Can you work these out from the model? Positions are in its coordinate system, mm. Face numbers are marked on the shaded views. A direction names the side the tool comes from. Round coordinates to 2 decimals unless told otherwise and drop trailing zeros. Write each loop counter-clockwise with the first axis right and the second up, starting at its lowest first coordinate (ties: lowest second). Pieces come first, ordered by that corner, then holes. Notation, with made-up numbers: M 69.5,82 L 95.5,82 A4 cw 95.5,88 Z; hole C 36,-20 d6. An arc over 180 degrees is marked long. Answer as a JSON object with one key per item and string values. Group by question number.
1) Suppose I cut it at C-C, the plane z = -9.5. Write out the boundary of the cut face in (x, y).
2) Suppose I cut it at B-B, the plane y = 0. State how many separate pieces and enclosed holes the cut face has, and give its area (3 significant figures).
3) Suppose I cut it at A-A, the plane z = -14.5. Write out the boundary of the cut face in (x, y).
4) If we mould it in two halves opening along X, with no side actions, what happens to the marked faces 4, 5 and 6? For each: +X half, -X half, draft (parallel to the pull), parting line (faces both ways), or undercut.
5) Please list where these lines run through material, in increasing order: L1, parallel to Y at x = 0, z = -21.25; L2, parallel to Z at x = 23, y = 13; L3, parallel to Y at x = -23.5, z = -29. Write a range as [from, to].
6) I'm going to push flat-ended pins straight in: pin 1 Ø8 at (x, y) = (0, 22.5) entering from +Z; pin 2 Ø1.5 at (x, z) = (-20, -5) entering from -Y; pin 3 Ø10 at (x, z) = (12.5, -9.5) entering from +Y; pin 4 Ø3 at (x, z) = (-2.5, -17.5) entering from +Y. Where does each tip first touch, or does it pass through?
7) On a 3-axis mill with a long thin cutter (end or side, diameter ignored), from which of +Z, -Z, +X, -X, +Y, -Y can I reach the whole of each face in a straight line? I mean the marked faces 1, 2 and 3. Say none if no direction works.
from build123d import *

# Parameters (mm, degrees)
SKETCH_1_R                   = 17.5
EXTRUDE_1_DEPTH              = 12
SKETCH_2_R                   = 29
EXTRUDE_2_DEPTH              = 20
SKETCH_3_R                   = 6.5
CUT_EXTRUDE_1_DEPTH          = 53.019227215
SKETCH_4_R                   = 11.05
CUT_EXTRUDE_2_DEPTH          = 27
CHAMFER_1_SIZE               = 1
HOLE_WIZARD_M5_1_D           = 5.8
HOLE_WIZARD_M5_1_CBORE_D     = 10
HOLE_WIZARD_M5_1_CBORE_DEPTH = 5


with BuildPart() as part:
    # 草图1 → 凸台-拉伸1 (new body)
    with BuildSketch(Plane.XY):
        Circle(SKETCH_1_R)
    extrude(amount=-EXTRUDE_1_DEPTH)

    # 草图2 → 凸台-拉伸2 (add)
    with BuildSketch(Plane(origin=(0, 0, -12), x_dir=(-1, 0, 0), z_dir=(0, 0, -1))):
        Circle(SKETCH_2_R)
    extrude(amount=EXTRUDE_2_DEPTH)

    # 草图3 → 切除-拉伸1 (cut, through all)
    with BuildSketch(Plane.XY):
        Circle(SKETCH_3_R)
    extrude(amount=-CUT_EXTRUDE_1_DEPTH, mode=Mode.SUBTRACT)

    # 草图4 → 切除-拉伸2 (cut)
    with BuildSketch(Plane(origin=(0, 0, -32), x_dir=(-1, 0, 0), z_dir=(0, 0, -1))):
        Circle(SKETCH_4_R)
    extrude(amount=-CUT_EXTRUDE_2_DEPTH, mode=Mode.SUBTRACT)

    # 倒角1
    chamfer_1_edges = [part.edges().sort_by_distance(p)[0] for p in [
        (-17.5, 0, 0),
        (29, 0, -12),
        (29, 0, -32),
    ]]
    chamfer(chamfer_1_edges, length=CHAMFER_1_SIZE)

    # M5 六角凹头螺钉的柱形沉头孔1 (through all)
    with Locations(Plane(origin=(0, 0, -32), x_dir=(-1, 0, 0), z_dir=(0, 0, -1))):
        with Locations((0, 22.5), (-22.5, 0), (0, -22.5), (22.5, 0)):
            CounterBoreHole(HOLE_WIZARD_M5_1_D / 2, HOLE_WIZARD_M5_1_CBORE_D / 2, HOLE_WIZARD_M5_1_CBORE_DEPTH)


solid = part.part
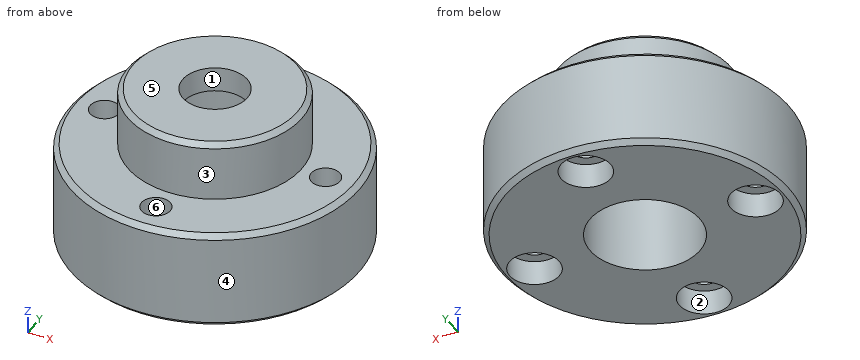
Results:
{
 "1": {"outline": "C 0,0 d35; hole C 0,0 d22.1"},
 "2": {"separate pieces": "4", "enclosed holes": "0", "area": "641 mm^2"},
 "3": {"outline": "C 0,0 d58; hole C -22.5,0 d5.8; hole C 0,0 d22.1; hole C 0,-22.5 d5.8; hole C 0,22.5 d5.8; hole C 22.5,0 d5.8"},
 "4": {"face 4": "parting line", "face 5": "draft", "face 6": "undercut"},
 "5": {"L1": "[-29, -25.4], [-19.6, -11.05], [11.05, 19.6], [25.4, 29]", "L2": "[-32, -12]", "L3": "[-16.99, -4.9], [4.9, 16.99]"},
 "6": {"pin 1": "z = -12", "pin 2": "through", "pin 3": "y = 27.59", "pin 4": "y = 28.98"},
 "7": {"face 1": "+Z, -Z", "face 2": "-Z", "face 3": "+Z"}
}
